Autodesk Inventor part; units mm, degrees
ref_plane "YZ Plane" through (0, 0, 0) normal (1, 0, 0) x (0, 1, 0)
ref_plane "XZ Plane" through (0, 0, 0) normal (0, 1, 0) x (-1, 0, 0)
ref_plane "XY Plane" through (0, 0, 0) normal (0, 0, 1) x (1, 0, 0)
sketch "Sketch_1" plane through (0, 0, 0) normal (0, 0, 1) x (1, 0, 0)
  line L0 (10, 0) -> (-2.8, 0)
  line L1 (-2.8, 0) -> (-2.8, 5)
  line L2 (-2.8, 5) -> (0, 5)
  line L3 (0, 5) -> (0, 3)
  line L4 (0, 3) -> (10, 3)
  line L5 (10, 3) -> (10, 0)
  line L6 (10, 0) -> (-2.8, 0)
revolve "Revolution1" add sketch "Sketch_1" angle 360 about axis through (10, 0, 0) along (1, 0, 0)
sketch "Sketch2" plane through (-2.8, 0, 0) normal (-1, 0, 0) x (0, 0, 1)
  point P0 (0, 0)
hole "Hole1" at (-2.8, 0, 0) direction (1, 0, 0) diameter 2.5 depth 2.5 tip angle 120
sketch "Sketch_3" plane through (-2.8, 0, 0) normal (1, 0, 0) x (0, 0, -1)
  line L0 (-1.25, -0.7217) -> (0, -1.4434)
  line L1 (0, -1.4434) -> (1.25, -0.7217)
  line L2 (1.25, -0.7217) -> (1.25, 0.7217)
  line L3 (1.25, 0.7217) -> (0, 1.4434)
  line L4 (0, 1.4434) -> (-1.25, 0.7217)
  line L5 (-1.25, 0.7217) -> (-1.25, -0.7217)
extrude "Extrusion1" cut sketch "Sketch_3" along normal blind 2.5
sketch "Sketch_6" plane through (0, 0, 0) normal (0, 0, 1) x (1, 0, 0)
  line L0 (14, 0) -> (10, 0)
  line L1 (10, 0) -> (10, 2)
  line L2 (10, 2) -> (13.5705, 2)
  line L3 (13.5705, 2) -> (14, 1.5705)
  line L4 (14, 1.5705) -> (14, 0)
  line L5 (14, 0) -> (10, 0)
revolve "Revolution2" add sketch "Sketch_6" angle 360 about axis through (14, 0, 0) along (1, 0, 0)
thread "Thread1"
properties part number "DBTS4-10-4"
Source: CAD feature listing. Evaluate the final solid. Frame: model axes, mm. A direction names the side the tool comes from. Coordinates: 2 decimals unless noted, no trailing zeros. Loops run counter-clockwise (first coordinate to the right, second up) from the corner with the lowest first, then second, coordinate; pieces in that order, holes last. Notation, with made-up numbers: (-19.5, -13) - (-7.5, -13) arc R16 cw to (-7.5, 9) - close; hole circle Ø4 at (13.5, 75). An arc over 180 degrees is marked (long way). Return JSON: item names as keys, results as strings.
Q1. Contact query for flat-ended pins moving along their axis: P1, Ø0.7, axis at x = -2, y = 0.5, coming from the +Z side; P2, Ø1.5, axis at x = 11.5, y = 2.5, coming from the -Z side; P3, Ø1, axis at x = 1, z = 1, coming from the +Y side. Output: stop coordinate, or through.
Results:
{"P1": "z = 5", "P2": "z = -0.97", "P3": "y = 2.96"}
Q2. Mould query, pull axis Z, two halves, no side actions, for faces 1 (the flat face through (14, 0, 0)), 2 (the conical face through (0.296, 0.065, 0.207)), 3 (the cylindrical face through (-1.38, -1.08, -4.88)). Classes: released by +Z, released by -Z, zero draft, split by the parting line, or undercut.
Results:
{"face 1": "zero draft", "face 2": "undercut", "face 3": "split by the parting line"}
Q3. Access query for faces 4 (the flat face through (-1.568, 1.088, 0.616)), 5 (the cylindrical face through (5, -3, 0)), 6 (the flat face through (-2.8, 1.04, -1.04)). Directions: +Z, -Z, +X, -X, +Y, -Y. A direction counts if a zero-diameter tool reaches every point of the face in a straight line with its end or side. Return the directions, or none.
Results:
{"face 4": "-X", "face 5": "+X", "face 6": "+Z, -Z, -X, +Y, -Y"}
Q4. Section B-B, the plane z = -2.5. Return loops of the section in (x, y).
Results:
{"outline": "(-2.8, -4.33) - (0, -4.33) - (0, -1.66) - (10, -1.66) - (10, 1.66) - (0, 1.66) - (0, 4.33) - (-2.8, 4.33) - close"}
Q5. Section D-D, the plane y = -3.75. Return loops of the section in (x, z).
Results:
{"outline": "(-2.8, -3.31) - (0, -3.31) - (0, 3.31) - (-2.8, 3.31) - close"}
Q6. Section C-C, the plane x = 5. Return loops of the section in (y, z), plus the area to 3 significant figures.
Results:
{"outline": "circle Ø6 at (0, 0)", "area": "28.3 mm2"}
Q7. Section A-A, the plane y = 2.25. Return loops of the section in (x, z).
Results:
{"outline": "(-2.8, -4.47) - (0, -4.47) - (0, -1.98) - (10, -1.98) - (10, 1.98) - (0, 1.98) - (0, 4.47) - (-2.8, 4.47) - close"}
Q8. Material intervals for line 1 along X through (y, z) = (-1.5, 3.5); line 2 along Y through (x, z) = (-0.25, -0.5); line 3 along X through (y, z) = (-2, -0.75), sorted ascending.
Results:
{"line 1": "-2.8 to 0", "line 2": "-4.97 to -1.05, 1.05 to 4.97", "line 3": "-2.8 to 10"}
